The model under review builds one solid part; all positions refer to its coordinate system, in mm. A direction names the side the tool comes from. Give positions to 0.01 mm unless a question says otherwise; leave off trailing zeros. Order: outer loops, then holes, each group sorted by start corner. A loop starts at its lowest first (then second) coordinate and runs counter-clockwise, first axis right, second up. Notation, with made-up numbers: (4.5, 8) - (30.5, 8) arc R20 ccw to (30.5, 23) - close; hole circle Ø6 at (-25.5, 21). An arc over 180 degrees is marked (long way). Use CSV: the item, a comma, the result in double quotes.
Autodesk Inventor part; units mm, degrees
ref_plane "YZ Plane" through (0, 0, 0) normal (1, 0, 0) x (0, 1, 0)
ref_plane "XZ Plane" through (0, 0, 0) normal (0, 1, 0) x (-1, 0, 0)
ref_plane "XY Plane" through (0, 0, 0) normal (0, 0, 1) x (1, 0, 0)
sketch "Sketch1" plane through (0, 0, 0) normal (0, 1, 0) x (-1, 0, 0)
  line L0 (7.031, 15.16) -> (-6.9736, 15.16)
  line L1 (6.9783, -15.1701) -> (7.031, 15.16)
  line L2 (7.031, 15.16) -> (-7.0217, -15.14) construction
  line L3 (-6.9736, 15.16) -> (6.9783, -15.1701) construction
  line L4 (-5.5, 10.15) -> (-3.5, 10.15) construction
  line L5 (6.9783, -15.1701) -> (4.0783, -15.1701)
  line L6 (4.0783, -15.1701) -> (4.0783, -7.6701)
  line L7 (-5.5, 10.15) -> (-4, 10.15) construction
  line L8 (1.5552, -10.543) -> (4.0783, -7.6701)
  line L9 (-6.9736, 15.16) -> (-6.9736, 9.96)
  line L10 (-6.9736, 9.96) -> (-5.4736, 9.96)
  line L11 (-5.4736, 9.96) -> (-4.4736, 10.96)
  line L12 (-5.4736, 9.96) -> (-4.0594, 9.96) construction
  line L13 (-4.4736, 10.96) -> (1.1832, 5.3031)
  line L14 (1.1832, 5.3031) -> (1.1832, -5.7347)
  line L15 (1.1832, -5.7347) -> (9.1832, -5.7347) construction
  line L16 (1.1832, -5.7347) -> (-3.6251, -10.543)
  line L17 (-3.6251, -10.543) -> (1.5552, -10.543)
  point P0 (0, 0)
  point P1 (-6.5, 10.15)
  dimension "d0" = 14
  dimension "d1" = 30.3
  dimension "d11" = 2.9
  dimension "d12" = 7.5
  dimension "d25" = 41.29
  dimension "d28" = 5.2
  dimension "d29" = 1.5
  dimension "d32" = 4.2
  dimension "d33" = 8
  dimension "d38" = 6.8
  dimension "d40" = 135
  dimension "d41" = 90
  dimension "d42" = 135
extrude "Extrusion1" add sketch "Sketch1" along normal blind 20
chamfer "Chamfer1" distance 2 angle 45 2 edges at (-7.031, 10, 15.16) (-6.9783, 10, -15.1701)
chamfer "Chamfer2" distance 1 angle 45 1 edges at (6.9736, 10, 15.16)
sketch "Sketch3" plane through (3.6251, 0, -10.543) normal (0, 0, -1) x (-1, 0, 0)
  line L0 (0, 0) -> (5.1803, 0) construction
  line L1 (5.1803, 0) -> (5.1803, 20) construction
  line L2 (0, 20) -> (5.1803, 20) construction
  line L3 (0, 0) -> (0, 20) construction
  line L4 (8.6561, 20) -> (-2.3485, 20) construction
  line L5 (5.1803, 0) -> (5.1803, 20) construction
  line L6 (5.1803, 10) -> (2.5543, 10) construction
  point P0 (3.6251, 0)
  dimension "d45" = 2.626
hole "Hole1" at (1.0708, 10, -10.543) direction (0, 0, 1) diameter 4 end through all
sketch "Sketch4" plane through (3.6251, 0, -10.543) normal (0, 0, -1) x (-1, 0, 0)
  circle A0 centre (2.5543, 10) radius 2 construction
  line L0 (2.5543, 8) -> (2.5543, 12)
  circle A1 centre (2.5543, 10) radius 2 construction
  line L1 (2.5543, 8) -> (0, 8)
  line L2 (0, 0) -> (0, 20)
  line L3 (0, 8) -> (0, 12)
  line L4 (0, 12) -> (2.5543, 12)
  point P0 (3.6251, 0)
extrude "Extrusion2" cut sketch "Sketch4" against normal blind 5
sketch "Sketch5" plane through (-5.031, 0, 15.16) normal (0, 0, 1) x (1, 0, 0)
  circle A0 centre (6.1018, 10) radius 2
  point P0 (5.031, 0)
hole "Hole2" at (1.0708, 10, 15.16) direction (0, 0, -1) diameter 8 depth 4
sketch "Sketch6" plane through (0, 20, 0) normal (0, 1, 0) x (1, 0, 0)
  line L0 (6.9736, -14.16) -> (5.9736, -15.16) construction
  line L1 (6.9736, -14.16) -> (6.9736, -9.96) construction
  line L2 (6.9736, -9.96) -> (5.4736, -9.96) construction
  line L3 (5.4736, -9.96) -> (4.4736, -10.96) construction
  line L4 (4.4736, -10.96) -> (-1.1832, -5.3031) construction
  line L5 (-1.1832, -5.3031) -> (-1.1832, 5.7347) construction
  line L6 (-1.1832, 5.7347) -> (3.6251, 10.543) construction
  line L7 (3.6251, 10.543) -> (-1.5552, 10.543) construction
  line L8 (-1.5552, 10.543) -> (-4.0783, 7.6701) construction
  line L9 (-4.0783, 7.6701) -> (-4.0783, 15.1701) construction
  line L10 (-4.0783, 15.1701) -> (-4.9783, 15.1701) construction
  line L11 (-6.9817, 13.1701) -> (-4.9783, 15.1701) construction
  line L12 (-6.9817, 13.1701) -> (-7.0275, -13.16) construction
  line L13 (-5.031, -15.16) -> (-7.0275, -13.16) construction
  line L14 (-5.031, -15.16) -> (5.9736, -15.16) construction
  line L15 (-6.9817, 13.1701) -> (-7.0275, -13.16) construction
  line L16 (-7.0275, -13.16) -> (-7.0046, 0.005) construction
  line L17 (-7.0046, 0.005) -> (-4.0046, -0.0002) construction
  line L18 (-4.0046, -0.0002) -> (-4.0046, 4.9998)
  line L19 (-4.0046, -0.0002) -> (0.9954, -0.0002) construction
  line L20 (-4.0046, -0.0002) -> (-4.0046, -5.0002)
  line L21 (-4.0046, -5.0002) -> (-7.0081, -1.9967)
  line L22 (-4.0046, 4.9998) -> (-7.0011, 2.0033)
  line L23 (-7.0081, -1.9967) -> (-7.0011, 2.0033)
  point P0 (0, 0)
  dimension "d63" = 13.165
  dimension "d64" = 3
  dimension "d65" = 5
  dimension "d66" = 90
  dimension "d67" = 5
  dimension "d68" = 45
  dimension "d69" = 45
extrude "Extrusion3" cut sketch "Sketch6" against normal through all
equation "\"d42\" = d40"
equation "\"d69\" = d68"
properties part number "bolt_part"
Item 1: Take a section at B-B, the plane x = -0.5. Give the boundary of the cut face in (y, z).
Results list:
outline,"(0, -10.54) - (8.76, -10.54) - (8.76, -6.42) - (0, -6.42) - close; (0, 5.99) - (8.76, 5.99) - (8.76, 11.16) - (6.32, 11.16) - (6.32, 15.16) - (0, 15.16) - close; (11.24, -10.54) - (20, -10.54) - (20, -6.42) - (11.24, -6.42) - close; (11.24, 5.99) - (20, 5.99) - (20, 15.16) - (13.68, 15.16) - (13.68, 11.16) - (11.24, 11.16) - close"
Item 2: Take a section at C-C, the plane z = -4. Give the boundary of the cut face in (x, y).
Results list:
outline,"(-7, 0) - (-5, 0) - (-5, 20) - (-7, 20) - close; (-4, 0) - (-1.18, 0) - (-1.18, 20) - (-4, 20) - close"
Item 3: Take a section at D-D, the plane x = -4.5. Give the boundary of the cut face in (y, z).
Results list:
outline,"(0, -15.17) - (20, -15.17) - (20, -4.5) - (0, -4.5) - close; (0, 4.5) - (20, 4.5) - (20, 15.16) - (0, 15.16) - close"
Item 4: Take a section at A-A, the plane y = 10. Give the boundary of the cut face in (x, z).
Results list:
outline,"(-7.03, 13.16) - (-7.01, 2) - (-4, 5) - (-4, -5) - (-7, -2) - (-6.98, -13.17) - (-4.98, -15.17) - (-4.08, -15.17) - (-4.08, -7.67) - (-1.56, -10.54) - (-0.93, -10.54) - (-0.93, -5.99) - (-1.18, -5.73) - (-1.18, 5.3) - (-0.93, 5.56) - (-0.93, 11.16) - (-2.93, 11.16) - (-2.93, 15.16) - (-5.03, 15.16) - close; (3.07, 9.56) - (4.47, 10.96) - (5.47, 9.96) - (6.97, 9.96) - (6.97, 14.16) - (5.97, 15.16) - (5.07, 15.16) - (5.07, 11.16) - (3.07, 11.16) - close"
Item 5: Clearance check with flat-ended pins moving along their axes: pin 1 (2 mm diameter, centred on y = 7, z = -10, fed in from +X); pin 2 (2.5 mm diameter, centred on x = 2, y = 7, fed in from -Z); pin 3 (1.3 mm diameter, centred on x = 2.5, z = -10, fed in from -Y); pin 4 (11 mm diameter, centred on y = 14.5, z = -0.5, fed in from -X). State where each tip first meets the part, or that it passes through.
Results list:
pin 1,"stops at x = 3.63"
pin 2,"stops at z = -10.54"
pin 3,"stops at y = 0"
pin 4,"stops at x = -7.01"
Item 6: Mouldability with a two-part tool opening along Z and no side actions: class faces 1 (the face through (-4.005, 10, 0)), 2 (the face through (6.974, 10, 12)), 3 (the face through (6, 10, 9.96)), 4 (the face through (6.481, 10.14, 14.653)) as pulls with the +Z half, pulls with the -Z half, needs draft (parallel to the pull), parting line crosses it, or undercut.
Results list:
face 1,"undercut"
face 2,"needs draft"
face 3,"pulls with the -Z half"
face 4,"pulls with the +Z half"
Item 7: Wall thickness on L1, parallel to Z at x = 3, y = 5.5; L2, parallel to Z at x = -0.25, y = 3.5; L3, parallel to X at y = 5, z = 3: over which ranges is each line inside the solid? List them lowest first.
Results list:
L1,"z = -10.54 to -9.92, 9.49 to 15.16"
L2,"z = -10.54 to -6.67, 6.24 to 15.16"
L3,"x = -7.01 to -6, -4 to -1.18"
Item 8: Tool access review of faces 5 (the face through (1.19, 7.64, -8.11)), 6 (the face through (-5.485, 10.14, 3.519)), 7 (the face through (-4.078, 10, -11)): name each direction out of +Z, -Z, +X, -X, +Y, -Y from which nothing blocks a thin tool from reaching the whole face with its end or side.
Results list:
face 5,"+X, +Y, -Y"
face 6,"+Y, -Y"
face 7,"-Z, +Y, -Y"
